from build123d import *

# Parameters (mm, degrees)
SKETCH1_W           = 40
SKETCH1_H           = 20
BOSS_EXTRUDE1_DEPTH = 5
SKETCH2_W           = 3
SKETCH2_H           = 20
BOSS_EXTRUDE2_DEPTH = 30
SKETCH3_W           = 5
SKETCH3_H           = 20
BOSS_EXTRUDE3_DEPTH = 45
SKETCH4_W           = 5
SKETCH4_H           = 20
BOSS_EXTRUDE4_DEPTH = 30
SKETCH5_W           = 34
SKETCH5_H           = 20
BOSS_EXTRUDE5_DEPTH = 2
SKETCH6_R           = 7.5
CUT_EXTRUDE1_DEPTH  = 2
SKETCH7_R           = 5.085514488
CUT_EXTRUDE2_DEPTH  = 5
SKETCH8_R           = 6.5
CUT_EXTRUDE3_DEPTH  = 13


with BuildPart() as part:
    # Sketch1 → Boss-Extrude1 (new body)
    with BuildSketch(Plane.XY):
        Rectangle(SKETCH1_W, SKETCH1_H)
    extrude(amount=BOSS_EXTRUDE1_DEPTH)

    # Sketch2 → Boss-Extrude2 (add)
    with BuildSketch(Plane.XY.offset(5)):
        with Locations((-18.5, 0)):
            Rectangle(SKETCH2_W, SKETCH2_H)
        with Locations((18.5, 0)):
            Rectangle(SKETCH2_W, SKETCH2_H)
    extrude(amount=BOSS_EXTRUDE2_DEPTH)

    # Sketch3 → Boss-Extrude3 (add)
    with BuildSketch(Plane(origin=(20, 0, 0), x_dir=(0, 0, -1), z_dir=(1, 0, 0))):
        with Locations((-32.5, 0)):
            Rectangle(SKETCH3_W, SKETCH3_H)
    extrude(amount=BOSS_EXTRUDE3_DEPTH)

    # Sketch4 → Boss-Extrude4 (add)
    with BuildSketch(Plane.ZY.offset(20)):
        with Locations((32.5, 0)):
            Rectangle(SKETCH4_W, SKETCH4_H)
    extrude(amount=BOSS_EXTRUDE4_DEPTH)

    # Sketch5 → Boss-Extrude5 (add)
    with BuildSketch(Plane.XY.offset(35)):
        Rectangle(SKETCH5_W, SKETCH5_H)
    extrude(amount=-BOSS_EXTRUDE5_DEPTH)

    # Sketch6 → Cut-Extrude1 (cut)
    with BuildSketch(Plane(origin=(0, 0, 0), x_dir=(-1, 0, 0), z_dir=(0, 0, -1))):
        Circle(SKETCH6_R)
    extrude(amount=-CUT_EXTRUDE1_DEPTH, mode=Mode.SUBTRACT)

    # Sketch7 → Cut-Extrude2 (cut)
    with BuildSketch(Plane(origin=(0, 0, 2), x_dir=(-1, 0, 0), z_dir=(0, 0, -1))):
        Circle(SKETCH7_R)
    extrude(amount=-CUT_EXTRUDE2_DEPTH, mode=Mode.SUBTRACT)

    # Sketch8 → Cut-Extrude3 (cut)
    with BuildSketch(Plane.XY.offset(35)):
        Circle(SKETCH8_R)
    extrude(amount=-CUT_EXTRUDE3_DEPTH, mode=Mode.SUBTRACT)


solid = part.part
Source: CAD feature listing. Evaluate the final solid. Frame: model axes, mm. A direction names the side the tool comes from. Coordinates: 2 decimals unless noted, no trailing zeros. Loops run counter-clockwise (first coordinate to the right, second up) from the corner with the lowest first, then second, coordinate; pieces in that order, holes last. Notation, with made-up numbers: (-15, 49) - (37, 49) arc R5 cw to (37, 55) - close; hole circle Ø8 at (18, -17.75). An arc over 180 degrees is marked (long way). Return JSON: item names as keys, results as strings.
Q1. Section C-C, the plane x = 0. Return loops of the section in (y, z).
Results:
{"outline": "(-10, 0) - (-7.5, 0) - (-7.5, 2) - (-5.09, 2) - (-5.09, 5) - (-10, 5) - close; (-10, 33) - (-6.5, 33) - (-6.5, 35) - (-10, 35) - close; (5.09, 2) - (7.5, 2) - (7.5, 0) - (10, 0) - (10, 5) - (5.09, 5) - close; (6.5, 33) - (10, 33) - (10, 35) - (6.5, 35) - close"}
Q2. Contact query for flat-ended pins moving along their axis: P1, Ø9, axis at x = 0, y = 0, coming from the -Z side; P2, Ø10, axis at y = -5, z = 15.5, coming from the +X side; P3, Ø10, axis at x = -36, y = -3.5, coming from the -Z side; P4, Ø10.5, axis at x = 0, y = 0, coming from the +Z side. Output: stop coordinate, or through.
Results:
{"P1": "through", "P2": "x = 20", "P3": "z = 30", "P4": "z = 5"}
Q3. Material intervals for line 1 along X through (y, z) = (-8.75, 26.5); line 2 along Y through (x, z) = (0, 34.2); line 3 along X through (y, z) = (-8.75, 30.5), sorted ascending.
Results:
{"line 1": "-20 to -17, 17 to 20", "line 2": "-10 to -6.5, 6.5 to 10", "line 3": "-50 to -17, 17 to 65"}
Q4. Mould query, pull axis Y, two halves, no side actions, for faces 1 (the flat face through (42, 0, 30)), 2 (the cylindrical face through (7.493, 0.33, 0.986)), 3 (the flat face through (-1, -10, 34)). Classes: released by +Y, released by -Y, zero draft, split by the parting line, or undercut.
Results:
{"face 1": "zero draft", "face 2": "undercut", "face 3": "released by -Y"}
Q5. Access query for faces 4 (the flat face through (-20, 0, 15)), 5 (the flat face through (0, 7, 33)), 6 (the flat face through (20, 0, 15)). Directions: +Z, -Z, +X, -X, +Y, -Y. A direction counts if a zero-diameter tool reaches every point of the face in a straight line with its end or side. Return the directions, or none.
Results:
{"face 4": "-Z, -X, +Y, -Y", "face 5": "+Y, -Y", "face 6": "-Z, +X, +Y, -Y"}
Q6. Section D-D, the plane z = 16. Return loops of the section in (x, y), plus the area to 3 significant figures.
Results:
{"outline": "(-20, -10) - (-17, -10) - (-17, 10) - (-20, 10) - close; (17, -10) - (20, -10) - (20, 10) - (17, 10) - close", "area": "120 mm2"}
Q7. Section A-A, the plane y = 0. Return loops of the section in (x, z).
Results:
{"outline": "(-50, 30) - (-20, 30) - (-20, 0) - (-7.5, 0) - (-7.5, 2) - (-5.09, 2) - (-5.09, 5) - (-17, 5) - (-17, 33) - (-6.5, 33) - (-6.5, 35) - (-50, 35) - close; (5.09, 2) - (7.5, 2) - (7.5, 0) - (20, 0) - (20, 30) - (65, 30) - (65, 35) - (6.5, 35) - (6.5, 33) - (17, 33) - (17, 5) - (5.09, 5) - close"}
Q8. Section B-B, the plane z = 31. Return loops of the section in (x, y), plus the area to 3 significant figures.
Results:
{"outline": "(-50, -10) - (-17, -10) - (-17, 10) - (-50, 10) - close; (17, -10) - (65, -10) - (65, 10) - (17, 10) - close", "area": "1,620 mm2"}
